Design review of the part built by this model. Coordinates are the model's own, in mm. Give positions to 0.01 mm unless a question says otherwise; leave off trailing zeros. Write each loop counter-clockwise with the first axis right and the second up, starting at its lowest first coordinate (ties: lowest second). Pieces come first, ordered by that corner, then holes. Notation, with made-up numbers: (16, 3.25) -> (23, 3.25) arc R34 ccw to (23, 41.25) -> close; hole circle Ø8 at (43, 85.25). An arc over 180 degrees is marked (long way). Answer as a JSON object with one key per item and string values.
```python
from build123d import *

# Parameters (mm, degrees)
F0_W     = 50.8
F0_H     = 50.8
F1_DEPTH = 50.8
F4_DEPTH = 50.8


with BuildPart() as f1:
    # F0 (on Front) → F1 (new body)
    with BuildSketch(Plane.XZ):
        with Locations((25.4, 25.4)):
            Rectangle(F0_W, F0_H)
    extrude(amount=F1_DEPTH)

    # F2 (on face) → F4 (cut)
    with BuildSketch(Plane.XZ.offset(50.8)):
        with BuildLine():
            Line((0, 50.8), (0, 25.4))
            ThreePointArc((0, 25.4), (18.682128, 32.117872), (25.4, 50.8))
            Line((25.4, 50.8), (0, 50.8))
        make_face()
    extrude(amount=-F4_DEPTH, mode=Mode.SUBTRACT)


solid = f1.part
```
(1) We need section A-A, the plane y = -13. State the section outline as (x, z) points (3 decimals), then the cut area to 3 significant figures.
Here are the results:
{"outline": "(0, 0) -> (50.8, 0) -> (50.8, 50.8) -> (25.4, 50.8) arc R23.295 cw to (0, 25.4) -> close", "area": "2,050 mm²"}
(2) We need section B-B, the plane x = 20. State the section outline as (y, z) points.
Here are the results:
{"outline": "(-50.8, 0) -> (0, 0) -> (0, 33.55) -> (-50.8, 33.55) -> close"}
(3) Clearance check with flat-ended pins moving along their axes: pin 1 (4 mm diameter, centred on x = 18.5, y = -30, fed in from +Z); pin 2 (1 mm diameter, centred on x = 23, y = -21.5, fed in from +Z) (3 decimals); pin 3 (5 mm diameter, centred on x = 21, z = 45.5, fed in from -Y). State where each tip first meets the part, or that it passes through.
Here are the results:
{"pin 1": "stops at z = 34.16", "pin 2": "stops at z = 39.135", "pin 3": "passes through"}
(4) For line 1 along X through (y, z) = (-26.5, 33); line 2 along Z through (x, y) = (6.5, -28); line 3 along Z through (x, y) = (4.5, -41), list the stretches that pass through material, from the lowest coordinate up.
Here are the results:
{"line 1": "x = 19.52 to 50.8", "line 2": "z = 0 to 25.69", "line 3": "z = 0 to 25.41"}
(5) We need section C-C, the plane z = 32. State the section outline as (x, y) points, then the cut area to 3 significant figures.
Here are the results:
{"outline": "(18.56, -50.8) -> (50.8, -50.8) -> (50.8, 0) -> (18.56, 0) -> close", "area": "1,640 mm²"}
